```python
from build123d import *

# Parameters (mm, degrees)
BOSS_EXTRUDE1_DEPTH  = 12.7
M4_CLEARANCE_HOLE1_D = 4.3


with BuildPart() as part:
    # Sketch1 → Boss-Extrude1 (new body)
    with BuildSketch(Plane.XY):
        Polygon((54.99, 29.865), (15.01, 29.865), (15.01, 19.865), (31.995, 19.865), (31.995, 22.86), (38.005, 22.86), (38.005, 19.865), (54.99, 19.865), align=None)
    extrude(amount=-BOSS_EXTRUDE1_DEPTH)

    # M4 Clearance Hole1 (through all)
    with Locations(Plane(origin=(25, 19.865, -6.35), x_dir=(0, 0, -1), z_dir=(0, -1, 0))):
        with Locations((0, 0), (0, 20)):
            Hole(M4_CLEARANCE_HOLE1_D / 2)


solid = part.part
```
Model file for the job. Use its own axes, mm. A direction names the side the tool comes from. Coordinates: 2 decimals unless noted, no trailing zeros. Order: outer loops, then holes, each group sorted by start corner. A loop starts at its lowest first (then second) coordinate and runs counter-clockwise, first axis right, second up. Notation, with made-up numbers: (69, 78.5) -> (100, 78.5) arc R19 cw to (100, 112.5) -> close; hole circle Ø7 at (3, -32). An arc over 180 degrees is marked (long way). Answer as a JSON object with one key per item and string values. Group by question number.
1) Cut at C-C, the plane x = 25. Write the cut outline in (y, z) (3 decimals), then the cut area to 3 significant figures.
2) Cut at A-A, the plane y = 21. Write the cut outline in (x, z) (3 decimals).
3) Pull direction Z, two halves, no side cores. Call faces 3 (the face through (38.005, 21, -6)), 4 (the face through (22.9, 24.94, -6.82)), 5 (the face through (35, 25, -12.7)): +Z half, -Z half, draft (parallel to the pull), parting line (faces both ways), or undercut.
4) Which spindle directions (+Z, -Z, +X, -X, +Y, -Y) get a long thin tool onto all of the face, cutting with end or side? Do faces 1 (the face through (35, 25, 0)), 2 (the face through (35, 22.86, -6)). Say none if no direction does.
5) Drill centre lines: L1, parallel to X at y = 24.5, z = -6.35; L2, parallel to X at y = 21.5, z = -3.5 (3 decimals). Where is each one in solid material? Low to high.
6) Cut at B-B, the plane z = -6.35. Write the cut outline in (x, y) (3 decimals).
7) Cut at D-D, the plane y = 25.5. Write the cut outline in (x, z), then the cut area to 3 significant figures.
8) Flat gauge pin, fed straight in: pin 1 (4 mm diameter, centred on x = 25, z = -6.35, fed in from -Y). Where does the tip first touch, or does it go through?
Check values:
{
 "1": {"outline": "(19.865, -12.7) -> (29.865, -12.7) -> (29.865, -8.5) -> (19.865, -8.5) -> close; (19.865, -4.2) -> (29.865, -4.2) -> (29.865, 0) -> (19.865, 0) -> close", "area": "84.0 mm²"},
 "2": {"outline": "(15.01, -12.7) -> (31.995, -12.7) -> (31.995, 0) -> (15.01, 0) -> close; (38.005, -12.7) -> (54.99, -12.7) -> (54.99, 0) -> (38.005, 0) -> close; hole circle Ø4.3 at (25, -6.35); hole circle Ø4.3 at (45, -6.35)"},
 "3": {"face 3": "draft", "face 4": "undercut", "face 5": "-Z half"},
 "4": {"face 1": "+Z, +X, -X, +Y, -Y", "face 2": "+Z, -Z, -Y"},
 "5": {"L1": "x = 15.01 to 22.85, 27.15 to 42.85, 47.15 to 54.99", "L2": "x = 15.01 to 31.995, 38.005 to 54.99"},
 "6": {"outline": "(15.01, 19.865) -> (22.85, 19.865) -> (22.85, 29.865) -> (15.01, 29.865) -> close; (27.15, 19.865) -> (31.995, 19.865) -> (31.995, 22.86) -> (38.005, 22.86) -> (38.005, 19.865) -> (42.85, 19.865) -> (42.85, 29.865) -> (27.15, 29.865) -> close; (47.15, 19.865) -> (54.99, 19.865) -> (54.99, 29.865) -> (47.15, 29.865) -> close"},
 "7": {"outline": "(15.01, -12.7) -> (54.99, -12.7) -> (54.99, 0) -> (15.01, 0) -> close; hole circle Ø4.3 at (25, -6.35); hole circle Ø4.3 at (45, -6.35)", "area": "479 mm²"},
 "8": {"pin 1": "passes through"}
}
